Design review of the part shown in the three views and the two pictorial views. Dimensions are in mm from the part's minimum x, y and z. A direction names the side the tool comes from. Give positions to 0.01 mm unless a question says otherwise; leave off trailing zeros. Write each loop counter-clockwise with the first axis right and the second up, starting at its lowest first coordinate (ties: lowest second). Pieces come first, ordered by that corner, then holes. Notation, with made-up numbers: M 31,2 L 89,2 A3 ccw 89,7 Z; hole C -13.5,16 d11. An arc over 180 degrees is marked long. Write item = value, one per line.
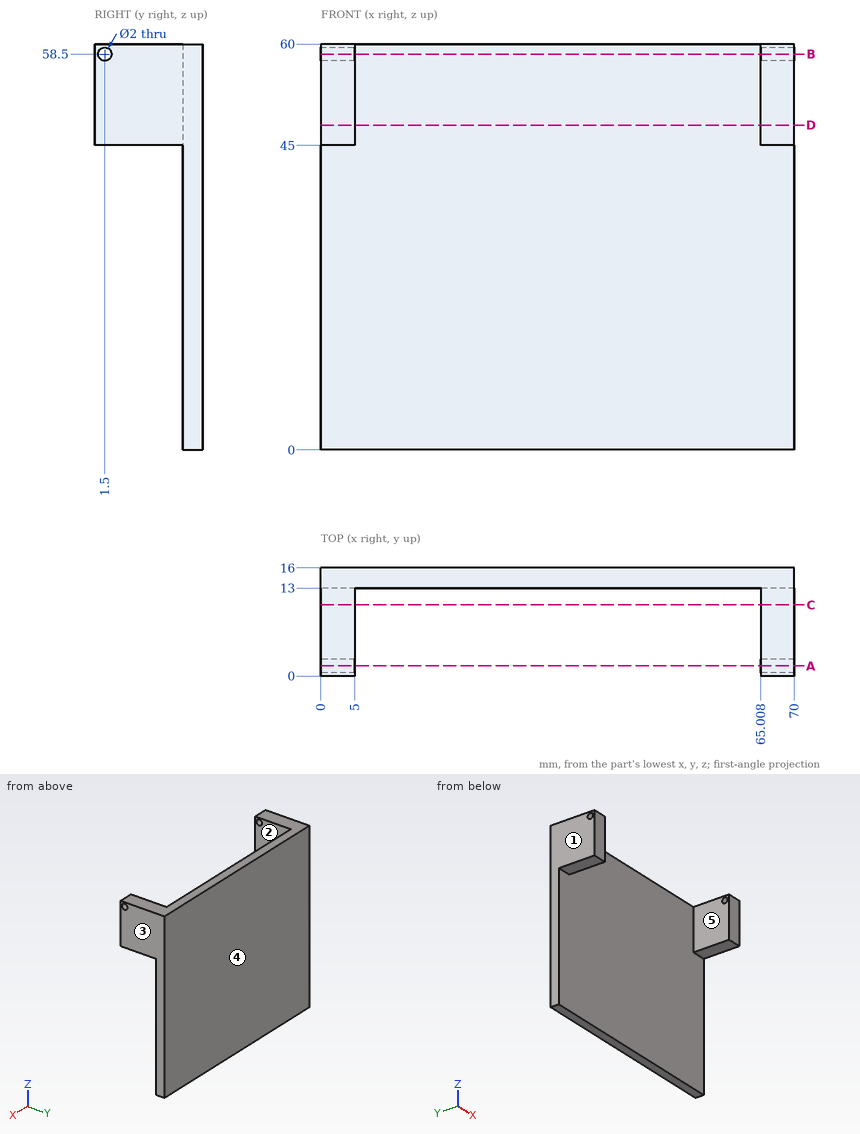
1. Machinability: for the marked faces 1 and 2, which of the approach directions +Z, -Z, +X, -X, +Y, -Y give a long, thin tool a straight path to every point of the face, cutting with its end or side? Answer none if there is none.
Responses:
face_1 = +Z, -Z, -X, +Y, -Y
face_2 = +Z, -Z, -Y
2. We need section C-C, the plane y = 10.5. Write out the cut boundary in (x, z), then the cut area to 3 significant figures.
Responses:
outline = M 0,45 L 5,45 L 5,60 L 0,60 Z; M 65.01,45 L 70,45 L 70,60 L 65.01,60 Z
area = 150 mm2
3. We need section B-B, the plane z = 58.5. Write out the cut boundary in (x, y), then the cut area to 3 significant figures.
Responses:
outline = M 0,0 L 5,0 L 5,0.5 L 0,0.5 Z; M 0,2.5 L 5,2.5 L 5,13 L 65.01,13 L 65.01,2.5 L 70,2.5 L 70,16 L 0,16 Z; M 65.01,0 L 70,0 L 70,0.5 L 65.01,0.5 Z
area = 320 mm2
4. We need section D-D, the plane z = 48. Write out the cut boundary in (x, y).
Responses:
outline = M 0,0 L 5,0 L 5,13 L 65.01,13 L 65.01,0 L 70,0 L 70,16 L 0,16 Z
5. We need section A-A, the plane y = 1.5. Write out the cut boundary in (x, z), then the cut area to 3 significant figures.
Responses:
outline = M 0,45 L 5,45 L 5,57.5 L 0,57.5 Z; M 0,59.5 L 5,59.5 L 5,60 L 0,60 Z; M 65.01,45 L 70,45 L 70,57.5 L 65.01,57.5 Z; M 65.01,59.5 L 70,59.5 L 70,60 L 65.01,60 Z
area = 130 mm2
6. The part is to be moulded in two halves that separate along X. For the marked faces 3, 4 and 5, say which applies: +X half, -X half, draft (parallel to the pull), parting line (faces both ways), or undercut.
Responses:
face_3 = +X half
face_4 = draft
face_5 = undercut
7. Insertion check: P1, Ø4, axis at x = 2.5, y = 5.5, coming from the -Z side; P2, Ø3, axis at x = 32, y = 10.5, coming from the +Z side. Each pin has a flat end and moves straight along its axis. Give the tip position at first contact, or say it passes through.
Responses:
P1 = 45
P2 = through
8. For line 1 along Y through (x, z) = (3.8, 58.5); line 2 along X through (y, z) = (4.75, 52.5); line 3 along Y through (x, z) = (1, 58), list the stretches that pass through material, from the lowest coordinate up. Write a range as from..to.
Responses:
line_1 = 0..0.5, 2.5..16
line_2 = 0..5, 65.01..70
line_3 = 0..0.63, 2.37..16
